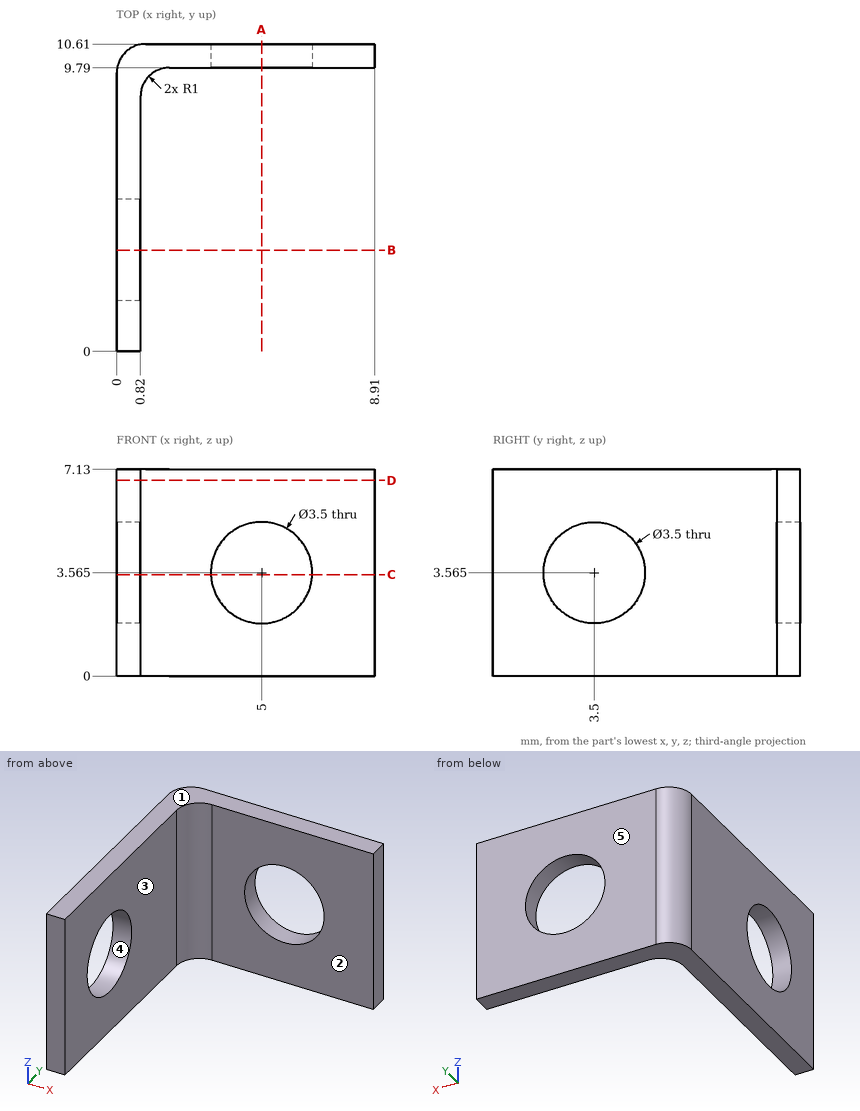
Job drawing, mm, ordinate dimensions from the low corner. One solid piece. A direction names the side the tool comes from. Coordinates: 2 decimals unless noted, no trailing zeros. Order: outer loops, then holes, each group sorted by start corner. A loop starts at its lowest first (then second) coordinate and runs counter-clockwise, first axis right, second up. Notation, with made-up numbers: (25, -7.5) - (55, -7.5) arc R22 cw to (55, 9.5) - close; hole circle Ø11 at (46, 79.5). An arc over 180 degrees is marked (long way). Return JSON: item names as keys, results as strings. Group by question number.
1) Saw through at C-C, the plane z = 3.5. Write the cut outline in (x, y).
2) Saw through at B-B, the plane y = 3.5. Write the cut outline in (x, z) (3 decimals), plus the area to 3 significant figures.
3) Mould opens along Y. For the marked faces 3, 4 and 5 say: released by +Y, released by -Y, zero draft, split by the parting line, or undercut.
4) Saw through at A-A, the plane x = 5. Write the cut outline in (y, z) (3 decimals), plus the area to 3 significant figures.
5) Flat gauge pins, fed straight in: P1, Ø3.5, axis at x = 6.5, z = 3.5, coming from the -Y side; P2, Ø2, axis at y = 4, z = 5, coming from the +X side. Where does each tip first touch, or does it go through?
6) Saw through at D-D, the plane z = 6.75. Write the cut outline in (x, y), plus the area to 3 significant figures.
7) Tool access for the marked faces 1 and 2: list every direction of +Z, -Z, +X, -X, +Y, -Y with a clear straight run to the whole face (end or side of a thin tool).
8) Probe line 1 (Z direction, x = 5, y = 10) (3 decimals); line 2 (Y direction, x = 8.25, z = 4.5); line 3 (Y direction, x = 0.75, z = 5). List the from-to ranges inside material, lowest first. Write a range as from..to.
Values found:
{
 "1": {"outline": "(0, 0) - (0.82, 0) - (0.82, 1.75) - (0, 1.75) - close; (0, 5.25) - (0.82, 5.25) - (0.82, 8.79) arc R1 cw to (1.82, 9.79) - (3.25, 9.79) - (3.25, 10.61) - (1, 10.61) arc R1 ccw to (0, 9.61) - close; (6.75, 9.79) - (8.91, 9.79) - (8.91, 10.61) - (6.75, 10.61) - close"},
 "2": {"outline": "(0, 0) - (0.82, 0) - (0.82, 1.815) - (0, 1.815) - close; (0, 5.315) - (0.82, 5.315) - (0.82, 7.13) - (0, 7.13) - close", "area": "2.98 mm²"},
 "3": {"face 3": "zero draft", "face 4": "undercut", "face 5": "released by +Y"},
 "4": {"outline": "(9.79, 0) - (10.61, 0) - (10.61, 1.815) - (9.79, 1.815) - close; (9.79, 5.315) - (10.61, 5.315) - (10.61, 7.13) - (9.79, 7.13) - close", "area": "2.98 mm²"},
 "5": {"P1": "stops at y = 9.79", "P2": "stops at x = 0.82"},
 "6": {"outline": "(0, 0) - (0.82, 0) - (0.82, 8.79) arc R1 cw to (1.82, 9.79) - (8.91, 9.79) - (8.91, 10.61) - (1, 10.61) arc R1 ccw to (0, 9.61) - close", "area": "15.3 mm²"},
 "7": {"face 1": "+Z, +X, -X, +Y, -Y", "face 2": "+Z, -Z, +X, -Y"},
 "8": {"line 1": "z = 0..1.815, 5.315..7.13", "line 2": "y = 9.79..10.61", "line 3": "y = 0..2.5, 4.5..10.58"}
}
